```python
from build123d import *

# Parameters (mm, degrees)
F0_R           = 50
F1_DEPTH       = 40
F2_D           = 12.1
F3_W           = 50
F3_H           = 100
F4_DEPTH       = 40
F5_D           = 17.5
F5_CBORE_D     = 31.5
F5_CBORE_DEPTH = 20
F7_DEPTH       = 25
F8_SIZE        = 5
F9_SIZE        = 10
F10_R          = 10


# Not quite as in the source:
# - a feature names something its author has since deleted; it is built from what else it names


with BuildPart() as f1:
    # F0 (on Front) → F1 (new body)
    with BuildSketch(Plane.XZ):
        with BuildLine():
            Line((-100, 158.1762170792), (-100, 0))
            Line((-100, 0), (100, 0))
            Line((100, 0), (100, 158.1762170792))
            ThreePointArc((100, 158.1762170792), (0, 58.1762170792), (-100, 158.1762170792))
        make_face()
        Polygon((-100, -40), (0, -40), (100, -40), (100, 0), (-100, 0), align=None)
        with BuildLine():
            ThreePointArc((100, 158.1762170792), (0, 258.1762170792), (-100, 158.1762170792))
            ThreePointArc((-100, 158.1762170792), (0, 58.1762170792), (100, 158.1762170792))
        make_face()
        with Locations((0, 158.1762170792)):
            Circle(F0_R, mode=Mode.SUBTRACT)
    extrude(amount=-F1_DEPTH)

    # F2 (through all)
    with Locations(Plane.XZ):
        with Locations((-72, 158.1762170792), (0, 230.1762170792), (71.9880287234, 159.4891224521), (0, 86.1762170792)):
            Hole(F2_D / 2)

    # F3 (on Top) → F4 (join)
    with BuildSketch(Plane.XY):
        Polygon((-25, 40), (-100, 40), (-100, -220), (-100, -260), (100, -260), (100, -220), (100, 40), (25, 40), (25, -60), (-25, -60), align=None)
        with Locations((0, -10)):
            Rectangle(F3_W, F3_H)
    extrude(amount=-F4_DEPTH)

    # F5 (through all)
    with Locations(Plane.XY):
        with Locations((-60, -100), (60, -100), (60, -220), (-60, -220)):
            CounterBoreHole(F5_D / 2, F5_CBORE_D / 2, F5_CBORE_DEPTH)

    # F6 (on Right) → F7 (join, symmetric)
    with BuildSketch(Plane.YZ):
        Polygon((-60, 0), (0, 0), (0, 60), align=None)
    extrude(amount=F7_DEPTH, both=True)

    # F8
    f8_edges = [f1.edges().sort_by_distance(p)[0] for p in [
        (-50, 0, 158.176217),
        (-50, 40, 158.176217),
    ]]
    chamfer(f8_edges, length=F8_SIZE)

    # F9
    f9_edges = [f1.edges().sort_by_distance(p)[0] for p in [
        (0, 40, -40),
        (-100, -260, -20),
        (100, -260, -20),
    ]]
    chamfer(f9_edges, length=F9_SIZE)

    # F10
    f10_edges = [f1.edges().sort_by_distance(p)[0] for p in [
        (-62.5, 0, 0),
        (62.5, 0, 0),
    ]]
    fillet(f10_edges, radius=F10_R)


solid = f1.part
```
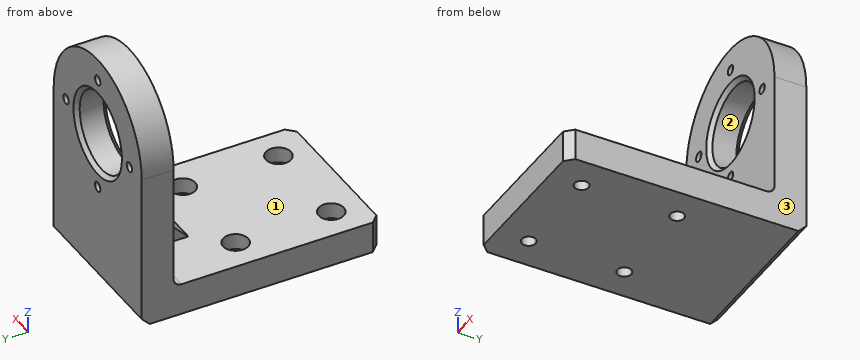
Model file for the job. Use its own axes, mm. Face numbers are marked on the shaded views. Coordinates: 2 decimals unless noted, no trailing zeros. Write each loop counter-clockwise with the first axis right and the second up, starting at its lowest first coordinate (ties: lowest second). Pieces come first, ordered by that corner, then holes. Notation, with made-up numbers: (72, 40.5) - (84, 40.5) arc R11 cw to (84, 57.5) - close; hole circle Ø2 at (-23, 6.25). An arc over 180 degrees is marked (long way). Use a Markdown table: item, result. Add a question column.
Item 1: Band-saw the part on A-A, the plane x = 0. Write the cut outline in (y, z).
Item 2: Drill centre lines: line 1 along Z through (x, y) = (0, 12.5); line 2 along Y through (x, z) = (60, -28.25); line 3 along Y through (x, z) = (60, -35.5). Where is each one in solid material? Low to high.
Item 3: Band-saw the part on B-B, the plane y = -220. Write the cut outline in (x, z), and give its area (3 significant figures).
Item 4: Band-saw the part on D-D, the plane z = 31.5. Write the cut outline in (x, y), and give its area (4 significant figures).
Item 5: Band-saw the part on C-C, the plane x = -60. Write the cut outline in (y, z).
Item 6: Drop flat-ended pins along their axis: pin 1 (20 mm diameter, centred on x = -60, y = -220, fed in from +Z); pin 2 (19.5 mm diameter, centred on x = 0, z = 86.18, fed in from -Y); pin 3 (25 mm diameter, centred on x = -67.5, y = -217, fed in from +Z). Give the stop position or say it passes through.
Item 7: Two-plate mould, pull along Z, no slides. Class the marked faces 1, 2 and 3: pulls with the +Z half, pulls with the -Z half, needs draft (parallel to the pull), parting line crosses it, or undercut.
A:
| question | item | result |
|---|---|---|
| 1 | outline | (-260, -40) - (30, -40) - (40, -30) - (40, 80.13) - (0, 80.13) - (0, 60) - (-60, 0) - (-260, 0) - close; (0, 92.23) - (40, 92.23) - (40, 103.18) - (35, 108.18) - (5, 108.18) - (0, 103.18) - close; (0, 213.18) - (5, 208.18) - (35, 208.18) - (40, 213.18) - (40, 224.13) - (0, 224.13) - close; (0, 236.23) - (40, 236.23) - (40, 258.18) - (0, 258.18) - close |
| 2 | line 1 | z = -40 to 80.13, 92.23 to 108.18, 208.18 to 224.13, 236.23 to 258.18 |
| 2 | line 2 | y = -260 to -228.75, -211.25 to -108.75, -91.25 to 40 |
| 2 | line 3 | y = -260 to -228.75, -211.25 to -108.75, -91.25 to 34.5 |
| 3 | outline | (-100, -40) - (-68.75, -40) - (-68.75, -20) - (-75.75, -20) - (-75.75, 0) - (-100, 0) - close; (-51.25, -40) - (51.25, -40) - (51.25, -20) - (44.25, -20) - (44.25, 0) - (-44.25, 0) - (-44.25, -20) - (-51.25, -20) - close; (68.75, -40) - (100, -40) - (100, 0) - (75.75, 0) - (75.75, -20) - (68.75, -20) - close |
| 3 | area | 6,040 mm² |
| 4 | outline | (-100, 0) - (-25, 0) - (-25, -28.5) - (25, -28.5) - (25, 0) - (100, 0) - (100, 40) - (-100, 40) - close |
| 4 | area | 9,425 mm² |
| 5 | outline | (-260, -40) - (-228.75, -40) - (-228.75, -20) - (-235.75, -20) - (-235.75, 0) - (-260, 0) - close; (-211.25, -40) - (-108.75, -40) - (-108.75, -20) - (-115.75, -20) - (-115.75, 0) - (-204.25, 0) - (-204.25, -20) - (-211.25, -20) - close; (-91.25, -40) - (30, -40) - (40, -30) - (40, 238.18) - (0, 238.18) - (0, 10) arc R10 cw to (-10, 0) - (-84.25, 0) - (-84.25, -20) - (-91.25, -20) - close |
| 6 | pin 1 | stops at z = -20 |
| 6 | pin 2 | stops at y = 0 |
| 6 | pin 3 | stops at z = 0 |
| 7 | face 1 | pulls with the +Z half |
| 7 | face 2 | undercut |
| 7 | face 3 | needs draft |
